Autodesk Inventor part; units mm, degrees
ref_plane "YZ Plane" through (0, 0, 0) normal (1, 0, 0) x (0, 1, 0)
ref_plane "XZ Plane" through (0, 0, 0) normal (0, 1, 0) x (-1, 0, 0)
ref_plane "XY Plane" through (0, 0, 0) normal (0, 0, 1) x (1, 0, 0)
sketch "Skizze1" plane through (0, 0, 0) normal (0, 0, 1) x (1, 0, 0)
  line L0 (0, 20) -> (10, 20)
  line L1 (10, 20) -> (10, 10.735)
  arc A0 (10, -10.735) -> (10, 10.735) centre (12.4, 0) ccw
  line L2 (0, 20) -> (0, -20)
  line L3 (0, -20) -> (10, -20)
  line L4 (10, -20) -> (10, -10.735)
  circle A1 centre (12.4, 0) radius 5.2
  point P0 (0, 0)
  dimension "d0" = 10
  dimension "d1" = 40
  dimension "d2" = 10
  dimension "d3" = 11
  dimension "d4" = 0
  dimension "d5" = 20
  dimension "d6" = 10.4
  dimension "d7" = 12.4
extrude "Extrusion1" add sketch "Skizze1" along normal blind 25
sketch "Skizze2" plane through (0, -20, 0) normal (-1, 0, 0) x (0, 0, 1)
  line L0 (0, 0) -> (25, 0)
  line L1 (0, 40) -> (5, 40)
  line L2 (5, 40) -> (5, 0)
  line L3 (5, 0) -> (0, 0)
  line L4 (0, 0) -> (0, 40)
  point P0 (0, 20)
  dimension "d10" = 5
extrude "Extrusion2" add sketch "Skizze2" along normal blind 20
sketch "Skizze3" plane through (0, 0, 0) normal (0, 0, -1) x (-1, 0, 0)
  circle A0 centre (10, -10) radius 1.6
  circle A1 centre (10, 10) radius 1.6
  line L0 (-10, -20) -> (20, -20)
  line L1 (20, 20) -> (20, -20)
  line L2 (20, 20) -> (-10, 20)
  point P0 (0, 0)
  dimension "d13" = 3.2
  dimension "d14" = 3.2
  dimension "d15" = 10
  dimension "d16" = 10
  dimension "d17" = 10
  dimension "d18" = 10
extrude "Extrusion3" cut sketch "Skizze3" against normal through all
fillet "Rundung1" radius 2 6 edges at (10, 20, 12.5) (10, 10.735, 12.5) (10, -10.735, 12.5) (10, -20, 12.5) (-20, -20, 2.5) (-20, 20, 2.5)
sketch "Skizze4" plane through (10, -18, 0) normal (1, 0, 0) x (0, 0, -1)
  circle A0 centre (-15, 3) radius 1.6
  circle A1 centre (-15, 33) radius 1.6
  line L0 (-25, -2) -> (0, -2)
  line L1 (-25, 0) -> (-25, 5.0062)
  line L2 (0, 38) -> (-25, 38)
  line L3 (-25, 30.9938) -> (-25, 36)
  point P0 (0, 18)
  dimension "d22" = 3.2
  dimension "d23" = 3.2
  dimension "d24" = 5
  dimension "d25" = 10
  dimension "d26" = 5
  dimension "d27" = 10
extrude "Extrusion4" cut sketch "Skizze4" against normal through all
sketch "Skizze5" plane through (0, 0, 25) normal (0, 0, 1) x (1, 0, 0)
  circle A0 centre (4.4, 0) radius 1.5
  circle A1 centre (12.4, 0) radius 5.2 construction
  circle A2 centre (12.4, -8) radius 1.5
  circle A3 centre (20.4, 0) radius 1.5
  circle A4 centre (12.4, 8) radius 1.5
  point P0 (0, 0)
  dimension "d30" = 3
  dimension "d31" = 8
  dimension "d34" = 360
extrude "Extrusion5" cut sketch "Skizze5" against normal blind 20
properties part number "Z nut mount" material "ABS-Kunststoff"
Source: CAD feature listing. Evaluate the final solid. Frame: model axes, mm. A direction names the side the tool comes from. Give positions to 0.01 mm unless a question says otherwise; leave off trailing zeros. Write each loop counter-clockwise with the first axis right and the second up, starting at its lowest first coordinate (ties: lowest second). Pieces come first, ordered by that corner, then holes.
1. Access query for faces 1 (the face through (9.4, -19.43, 12.68)), 2 (the face through (10, 16, 12)), 3 (the face through (4, 0, 5)). Directions: +Z, -Z, +X, -X, +Y, -Y. A direction counts if a zero-diameter tool reaches every point of the face in a straight line with its end or side. Return the directions, or none.
2. Section query C-C (z = 14). Return the cut outline in (x, y).
3. Pull-direction query (Y, two-part tool) for faces 4 (the face through (23.4, 0.2, 12.3)), 5 (the face through (-20, 0, 2)), 6 (the face through (12, 8, 5)), 7 (the face through (11.2, 7.1, 15.1)); classes: +Y half, -Y half, draft (parallel to the pull), parting line (faces both ways), or undercut.
4. Section query B-B (x = 9). Return the cut outline in (y, z).
5. Section query A-A (y = -15). Return the cut outline in (x, z).
6. Material intervals for line 1 along Y through (x, z) = (12.4, 9.25); line 2 along Y through (x, z) = (-10, 2.1); line 3 along X through (y, z) = (-14, 22.5), sorted ascending.
7. Section query D-D (x = 4.4). Return the cut outline in (y, z).
8. First-contact query: pin 1 (9.5 mm diameter, centred on x = 12.4, y = 0, fed in from -Z); pin 2 (3.5 mm diameter, centred on x = -10, y = 10, fed in from +Z); pin 3 (5 mm diameter, centred on y = -15, z = 15, fed in from -X); pin 4 (3 mm diameter, centred on x = 18.5, z = 6, fed in from +Y). Flat tips, straight axial feed; report the tip coordinate or a pass-through.
Output values:
1. face 1: +Z, -Z, +X, -Y
1. face 2: +Z, -Z, +X, +Y
1. face 3: +Z
2. outline: (0, -20) - (8, -20) arc R2 ccw to (10, -18) - (10, -16.25) - (0, -16.25) - close; (0, -13.75) - (10, -13.75) - (10, -12.99) arc R2 cw to (12.06, -10.99) arc R11 ccw (long way) to (12.06, 10.99) arc R2 cw to (10, 12.99) - (10, 13.75) - (0, 13.75) - close; (0, 16.25) - (10, 16.25) - (10, 18) arc R2 ccw to (8, 20) - (0, 20) - close; hole circle Ø3 at (4.4, 0); hole circle Ø10.4 at (12.4, 0); hole circle Ø3 at (12.4, -8); hole circle Ø3 at (12.4, 8); hole circle Ø3 at (20.4, 0)
3. face 4: parting line
3. face 5: draft
3. face 6: undercut
3. face 7: undercut
4. outline: (-19.73, 0) - (-3.93, 0) - (-3.93, 25) - (-19.73, 25) - close; (3.93, 0) - (19.73, 0) - (19.73, 25) - (3.93, 25) - close; hole circle Ø3.2 at (-15, 15); hole circle Ø3.2 at (15, 15)
5. outline: (-20, 0) - (10, 0) - (10, 13.4) - (0, 13.4) - (0, 5) - (-20, 5) - close; (0, 16.6) - (10, 16.6) - (10, 25) - (0, 25) - close
6. line 1: y = -11 to -9.5, -6.5 to -5.2, 5.2 to 6.5, 9.5 to 11
6. line 2: y = -20 to -11.6, -8.4 to 8.4, 11.6 to 20
6. line 3: x = 0 to 10
7. outline: (-20, 0) - (20, 0) - (20, 25) - (1.5, 25) - (1.5, 5) - (-1.5, 5) - (-1.5, 25) - (-20, 25) - close; hole circle Ø3.2 at (-15, 15); hole circle Ø3.2 at (15, 15)
8. pin 1: passes through
8. pin 2: stops at z = 5
8. pin 3: stops at x = 0
8. pin 4: stops at y = 9.99
